Work out the finished part from the listing and answer in its coordinate system (mm). A direction names the side the tool comes from. Give positions to 0.01 mm unless a question says otherwise; leave off trailing zeros. Order: outer loops, then holes, each group sorted by start corner. A loop starts at its lowest first (then second) coordinate and runs counter-clockwise, first axis right, second up. Notation, with made-up numbers: (61.5, 19.5) -> (78.5, 19.5) arc R25 cw to (78.5, 47.5) -> close; hole circle Ø5 at (69.25, 87.5). An arc over 180 degrees is marked (long way). Answer as CSV lines item,"result". Start each with the question number.
1. A cutting plane is placed at A-A (x = 48). Give the vertices of the cut face in (y, z).
2. A cutting plane is placed at D-D (z = -13). Give the vertices of the cut face in (x, y), then the cut area to 3 significant figures.
3. Flat-ended cylindrical pins translate along their axes: pin 1 (4.5 mm diameter, centred on x = -7, z = -32.5, fed in from +Y); pin 2 (4 mm diameter, centred on y = -60.5, z = 0, fed in from +X); pin 3 (11 mm diameter, centred on y = -27, z = -1.5, fed in from +X). Find the tip coordinate at first contact, or state that the pin passes through.
4. Find the intervals of material crossed by L1, parallel to Z at x = -2.35, y = -60.5; L2, parallel to X at y = -9, z = 2; L3, parallel to Y at x = 0, z = 0, in increasing order.
5. For faces 5 (the flat face through (-6, -20, -2)), 6 (the flat face through (7, -3, -9)), 7 (the cylindrical face through (1.617, -1.972, -0.67)), 8 (the flat face through (-4, -53, -9)), determine the directions among +Z, -Z, +X, -X, +Y, -Y from which every point of the face is accessible in a straight line to the end or side of a thin tool.
6. For a pull along Y with two mould halves and no side action, classify faces 1 (the flat face through (-6, -42, -27)), 2 (the cylindrical face through (-1.9, -58.75, 0.08)), 3 (the cylindrical face through (-6.34, -40.25, 0.08)), 4 (the flat face through (7, -3, 5)) as released by +Y, released by -Y, zero draft, split by the parting line, or undercut.
7. A cutting plane is placed at B-B (y = -60.5). Give the vertices of the cut face in (x, z), then the cut area to 3 significant figures.
8. A cutting plane is placed at C-C (z = 0). Give the vertices of the cut face in (x, y).
from build123d import *

# Parameters (mm, degrees)
F0_R     = 1.75
F1_DEPTH = 4
F4_DEPTH = 14
F6_DEPTH = 50.2
F5_R     = 1.75
F7_DEPTH = 71


# Not quite as in the source:
# - a feature names something its author has since deleted; it is built from what else it names


with BuildPart() as f1:
    # F0 (on Front) → F1 (new body)
    with BuildSketch(Plane.XZ):
        Polygon((-6, 5), (-6, 0), (-6, -9), (52, -9), (52, 0), (52, 5), align=None)
        Circle(F0_R, mode=Mode.SUBTRACT)
        with Locations((48, 0)):
            Circle(F0_R, mode=Mode.SUBTRACT)
    extrude(amount=F1_DEPTH)

    # F3 (on face) → F4 (join)
    with BuildSketch(Plane.XY.offset(5)):
        Polygon((-10, 0), (-10, -35), (-6, -35), (-6, -4), (-6, 0), align=None)
        Polygon((-6, -35), (-10, -35), (-9.275862069, -38), (-6, -38), align=None)
        Polygon((-5.275862069, -38), (-6, -35), (-6, -38), align=None)
        Polygon((-6, -38), (-9.275862069, -38), (-8.3103448276, -42), (-6, -42), align=None)
        Polygon((-4.3103448276, -42), (-5.275862069, -38), (-6, -38), (-6, -42), align=None)
        Polygon((-6, -42), (-8.3103448276, -42), (-6, -51.5714285714), align=None)
        Polygon((1, -64), (-4.3103448276, -42), (-6, -42), (-6, -51.5714285714), (-3, -64), align=None)
    extrude(amount=-F4_DEPTH)

    # F3 (on face) → F6 (join)
    with BuildSketch(Plane.XY.offset(5)):
        Polygon((-6, -38), (-9.275862069, -38), (-8.3103448276, -42), (-6, -42), align=None)
        Polygon((-4.3103448276, -42), (-5.275862069, -38), (-6, -38), (-6, -42), align=None)
    extrude(amount=-F6_DEPTH)

    # F5 (on face) → F7 (cut)
    with BuildSketch(Plane(origin=(-10, 0, 0), x_dir=(0, -1, 0), z_dir=(-1, 0, 0))):
        with Locations((42, 0)):
            Circle(F5_R)
        with Locations((60.5, 0)):
            Circle(F5_R)
    extrude(amount=-F7_DEPTH, mode=Mode.SUBTRACT)


solid = f1.part
Answer sheet:
1,outline,"(-4, -9) -> (0, -9) -> (0, -1.75) -> (-4, -1.75) -> close; (-4, 1.75) -> (0, 1.75) -> (0, 5) -> (-4, 5) -> close"
2,outline,"(-9.28, -38) -> (-8.31, -42) -> (-4.31, -42) -> (-5.28, -38) -> close"
2,area,"16.0 mm^2"
3,pin 1,"stops at y = -38"
3,pin 2,"stops at x = 0.64"
3,pin 3,"stops at x = -6"
4,L1,"z = -9 to -1.75, 1.75 to 5"
4,L2,"x = -10 to -6"
4,L3,"y = -64 to -62.25"
5,face 5,"+Z, -Z, +X"
5,face 6,"-Z, +X, -X, +Y"
5,face 7,"+Y"
5,face 8,"-Z, +X, -X, -Y"
6,face 1,"released by -Y"
6,face 2,"undercut"
6,face 3,"undercut"
6,face 4,"zero draft"
7,outline,"(-3.84, -9) -> (0.16, -9) -> (0.16, -1.75) -> (-3.84, -1.75) -> close; (-3.84, 1.75) -> (0.16, 1.75) -> (0.16, 5) -> (-3.84, 5) -> close"
7,area,"42.0 mm^2"
8,outline,"(-10, -35) -> (-8.73, -40.25) -> (-4.73, -40.25) -> (-6, -35) -> (-6, -4) -> (-1.75, -4) -> (-1.75, 0) -> (-10, 0) -> close; (-7.89, -43.75) -> (-4.27, -58.75) -> (-0.27, -58.75) -> (-3.89, -43.75) -> close; (-3.42, -62.25) -> (-3, -64) -> (1, -64) -> (0.58, -62.25) -> close; (1.75, -4) -> (46.25, -4) -> (46.25, 0) -> (1.75, 0) -> close; (49.75, -4) -> (52, -4) -> (52, 0) -> (49.75, 0) -> close"
